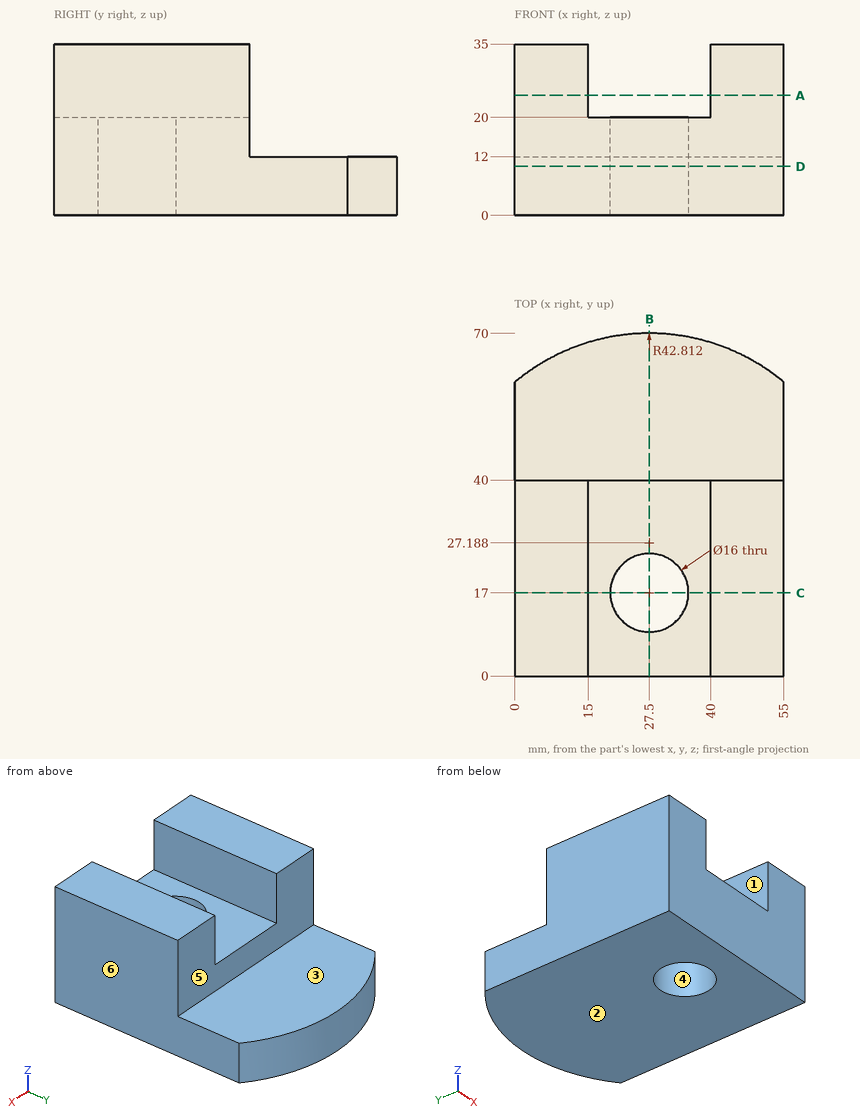
The drawing under review shows one solid part. Ordinate dimensions are in mm from its lowest x, y, z. A direction names the side the tool comes from. Coordinates: 2 decimals unless noted, no trailing zeros. Loops run counter-clockwise (first coordinate to the right, second up) from the corner with the lowest first, then second, coordinate; pieces in that order, holes last. Notation, with made-up numbers: M 69,-36 L 80,-36 A27 cw 80,-3 Z; hole C -7,15 d3. An arc over 180 degrees is marked long. Use one line per item in the form item = value.
(1) For the marked faces 1, 2 and 3, list the 3-axis set-ups (+Z, -Z, +X, -X, +Y, -Y) from which the entire face can be reached by the end or side of a thin tool; tool diameter is ignored.
Return value:
face_1 = +Z, +Y, -Y
face_2 = -Z, +X, -X, +Y, -Y
face_3 = +Z, +X, -X, +Y
(2) Consider section B-B (x = 27.5). Write out the cut boundary in (y, z).
Return value:
outline = M 0,0 L 9,0 L 9,20 L 0,20 Z; M 25,0 L 70,0 L 70,12 L 40,12 L 40,20 L 25,20 Z
(3) Clearance check with flat-ended pins moving along their axes: P1, Ø21, axis at x = 27.5, y = 17, coming from the -Z side; P2, Ø7, axis at x = 23, z = 19, coming from the +Y side. State where each tip first meets the part, or that it passes through.
Return value:
P1 = 0
P2 = 40
(4) Consider section D-D (z = 10). Write out the cut boundary in (x, y) (1 decimal).
Return value:
outline = M 0,0 L 55,0 L 55,60 A42.8 ccw 0,60 Z; hole C 27.5,17 d16
(5) For line 1 along Y through (x, z) = (27.5, 8); line 2 along X through (y, z) = (10, 28); line 3 along Y through (x, z) = (10, 20.5), list the stretches that pass through material, from the lowest coordinate up. Write a range as from..to.
Return value:
line_1 = 0..9, 25..70
line_2 = 0..15, 40..55
line_3 = 0..40
(6) Consider section A-A (z = 24.5). Write out the cut boundary in (x, y).
Return value:
outline = M 0,0 L 15,0 L 15,40 L 0,40 Z; M 40,0 L 55,0 L 55,40 L 40,40 Z
(7) Consider section C-C (y = 17). Write out the cut boundary in (x, z).
Return value:
outline = M 0,0 L 19.5,0 L 19.5,20 L 15,20 L 15,35 L 0,35 Z; M 35.5,0 L 55,0 L 55,35 L 40,35 L 40,20 L 35.5,20 Z
(8) Draft analysis for pull direction Y (two halves, no side actions). For the marked faces 4, 5 and 6, state which applies: pulls with the +Y half, pulls with the -Y half, needs draft (parallel to the pull), parting line crosses it, or undercut.
Return value:
face_4 = undercut
face_5 = pulls with the +Y half
face_6 = needs draft
